The listing builds one solid part. Answer for the finished solid, in the listing's coordinates (mm). A direction names the side the tool comes from. Coordinates: 2 decimals unless noted, no trailing zeros. Loops run counter-clockwise (first coordinate to the right, second up) from the corner with the lowest first, then second, coordinate; pieces in that order, holes last. Notation, with made-up numbers: (-22.75, -24) - (-5.75, -24) arc R24 ccw to (-5.75, 5) - close; hole circle Ø5 at (33, -8). An arc over 180 degrees is marked (long way). Return JSON: item names as keys, results as strings. Group by question number.
1. Find the intervals of material crossed by line 1 along Y through (x, z) = (3, -2.25); line 2 along Y through (x, z) = (0, 1); line 3 along X through (y, z) = (37, -2), in increasing order.
2. Each of these flat-tipped pins is pushed along its axis until it touches: P1, Ø3.5, axis at x = -0.5, z = -0.5, coming from the -Y side; P2, Ø0.5, axis at x = -0.5, y = 1.5, coming from the -Z side; P3, Ø2, axis at x = 0.5, y = 18.5, coming from the +Z side; P4, Ø3, axis at y = 21.5, z = 2, coming from the -X side. Where does it stop, or does it pass through?
3. The mould has two halves that part along Z. Classify faces 4 (the face through (-0.54, 23.54, -2.44)), 5 (the face through (0, 1, -1.5)), 6 (the face through (0, 2.5, 0)), 7 (the face through (0, 46.6, 0)): pulls with the +Z half, pulls with the -Z half, needs draft (parallel to the pull), parting line crosses it, or undercut.
4. Section B-B (y = 17) is taken. Write down the section's boundary in (x, z), and give its area (3 significant figures).
5. Which of the six approach directions +Z, -Z, +X, -X, +Y, -Y give full straight-line access (tool end or side, diameter ignored) to faces 1 (the face through (0, 0, -2)), 2 (the face through (1.293, 1.232, 0.76)), 3 (the face through (-2, 1.6, -2))?
6. Section A-A (x = 0) is taken. Write down the section's boundary in (y, z).
Autodesk Inventor part; units mm, degrees
ref_plane "YZ Plane" through (0, 0, 0) normal (1, 0, 0) x (0, 1, 0)
ref_plane "XZ Plane" through (0, 0, 0) normal (0, 1, 0) x (-1, 0, 0)
ref_plane "XY Plane" through (0, 0, 0) normal (0, 0, 1) x (1, 0, 0)
sketch "Boceto1" plane through (0, 0, 0) normal (0, 1, 0) x (-1, 0, 0)
  circle A0 centre (0, 0) radius 4.5
  dimension "d0" = 9
extrude "Extrusión1" add sketch "Boceto1" along normal blind 1.6
sketch "Boceto2" plane through (0, 1.6, 0) normal (0, 1, 0) x (1, 0, 0)
  circle A0 centre (0, 0) radius 2.5
  dimension "d3" = 5
extrude "Extrusión2" add sketch "Boceto2" along normal blind 45
fillet "Empalme1" radius 0.4 1 edges at (4.5, 0, 0)
fillet "Empalme2" radius 0.2 1 edges at (4.5, 1.6, 0)
sketch "Boceto3" plane through (0, 0, 0) normal (0, -1, 0) x (1, 0, 0)
  line L0 (-1.7321, 0) -> (-0.866, 1.5)
  line L1 (-0.866, 1.5) -> (0.866, 1.5)
  line L2 (0.866, 1.5) -> (1.7321, 0)
  line L3 (1.7321, 0) -> (0.866, -1.5)
  line L4 (0.866, -1.5) -> (-0.866, -1.5)
  line L5 (-0.866, -1.5) -> (-1.7321, 0)
  point P0 (0, 0)
  point P1 (0, 0)
  dimension "d8" = 3
extrude "Extrusión3" cut sketch "Boceto3" against normal blind 2.5
chamfer "Chaflán1" distance 0.5 angle 45 1 edges at (-2.5, 46.6, 0)
thread "Rosca2"
properties part number "Perno M5x8 cabeza plana" material "Hierro, gris"
The answers:
{
 "1": {"line 1": "y = 0 to 1.6", "line 2": "y = 2.5 to 46.6", "line 3": "x = -1.5 to 1.5"},
 "2": {"P1": "stops at y = 0", "P2": "stops at z = -4.49", "P3": "stops at z = 2.5", "P4": "stops at x = -2.45"},
 "3": {"face 4": "parting line crosses it", "face 5": "undercut", "face 6": "undercut", "face 7": "needs draft"},
 "4": {"outline": "circle Ø5 at (0, 0)", "area": "19.6 mm2"},
 "5": {"face 1": "+Z, -Z, +X, -X, -Y", "face 2": "-Y", "face 3": "+Y"},
 "6": {"outline": "(0, -4.1) arc R0.4 ccw to (0.4, -4.5) - (1.4, -4.5) arc R0.2 ccw to (1.6, -4.3) - (1.6, -2.5) - (46.1, -2.5) - (46.6, -2) - (46.6, 2) - (46.1, 2.5) - (1.6, 2.5) - (1.6, 4.3) arc R0.2 ccw to (1.4, 4.5) - (0.4, 4.5) arc R0.4 ccw to (0, 4.1) - (0, 1.5) - (2.5, 1.5) - (2.5, -1.5) - (0, -1.5) - close"}
}
